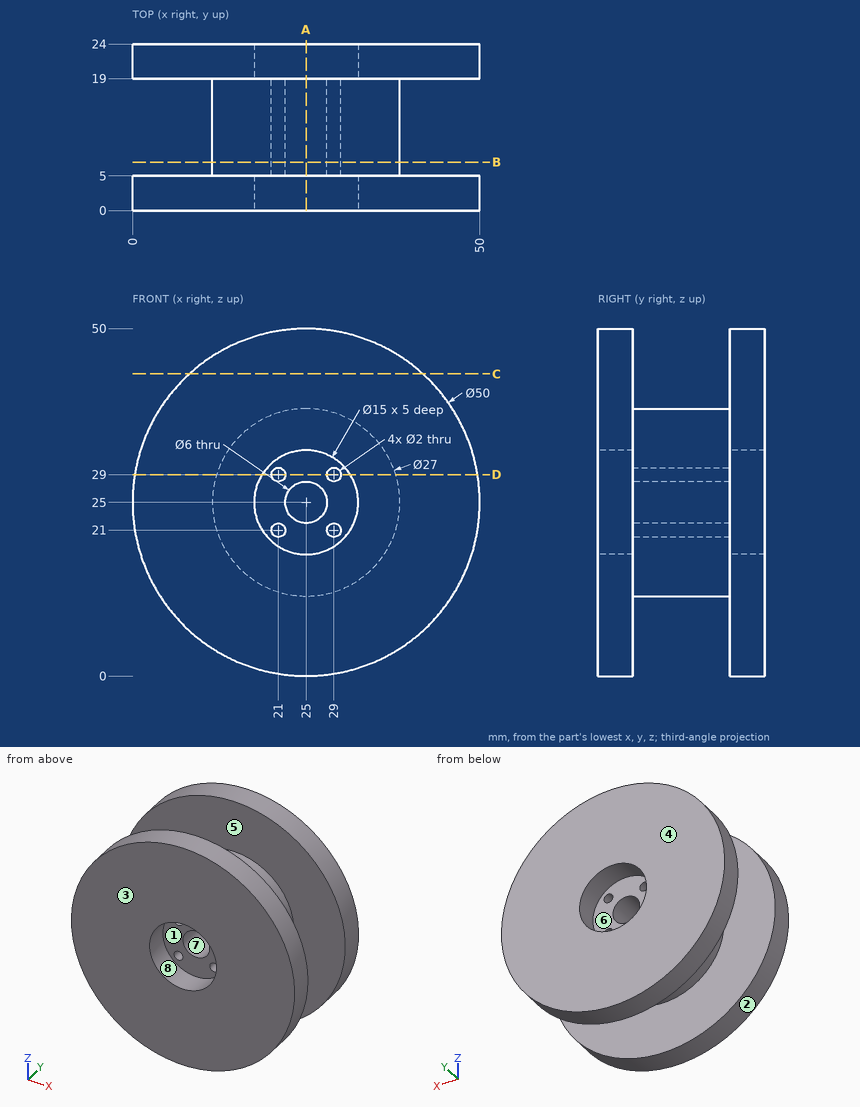
Design review of the part shown in the three views and the two pictorial views. Dimensions are in mm from the part's minimum x, y and z. A direction names the side the tool comes from. Round coordinates to 2 decimals unless told otherwise and drop trailing zeros. Order: outer loops, then holes, each group sorted by start corner. A loop starts at its lowest first (then second) coordinate and runs counter-clockwise, first axis right, second up.
Q1. Wall thickness on line 1 (Y direction, x = 38, z = 30); line 2 (X direction, y = 12.5, z = 25); line 3 (Z direction, x = 28.5, y = 12.25): over which ranges is each line inside the solid? List them lowest first.
Findings below:
line 1: y = 0 to 5, 19 to 24
line 2: x = 11.5 to 22, 28 to 38.5
line 3: z = 11.96 to 20.13, 21.87 to 28.13, 29.87 to 38.04
Q2. We need section B-B, the plane y = 7. Give the boundary of the cut face in (x, z).
Findings below:
outline: circle Ø27 at (25, 25); hole circle Ø2 at (21, 21); hole circle Ø2 at (21, 29); hole circle Ø6 at (25, 25); hole circle Ø2 at (29, 21); hole circle Ø2 at (29, 29)
Q3. We need section C-C, the plane z = 43.5. Give the boundary of the cut face in (x, y).
Findings below:
outline: (8.18, 0) - (41.82, 0) - (41.82, 5) - (8.18, 5) - close; (8.18, 19) - (41.82, 19) - (41.82, 24) - (8.18, 24) - close
Q4. Machinability: for the marked faces 4, 5, 6, 7 and 8, which of the approach directions +Z, -Z, +X, -X, +Y, -Y give a long, thin tool a straight path to every point of the face, cutting with its end or side? Answer none if there is none.
Findings below:
face 4: +Z, -Z, +X, -X, +Y
face 5: none
face 6: +Y
face 7: +Y, -Y
face 8: -Y
Q5. Mouldability with a two-part tool opening along X and no side actions: class the marked faces 1, 2 and 3 as pulls with the +X half, pulls with the -X half, needs draft (parallel to the pull), parting line crosses it, or undercut.
Findings below:
face 1: undercut
face 2: parting line crosses it
face 3: needs draft
Q6. Insertion check: P1, Ø3, axis at x = 20, z = 35, coming from the -Y side; P2, Ø8, axis at x = 10.5, y = 6, coming from the -Z side; P3, Ø2, axis at y = 14.5, z = 26, coming from the -X side; P4, Ø8, axis at x = 25, z = 25, coming from the +Y side. Each pin has a flat end and moves straight along its axis. Give the tip position at first contact, or say it passes through.
Findings below:
P1: stops at y = 0
P2: stops at z = 2.37
P3: stops at x = 11.5
P4: stops at y = 19
Q7. We need section A-A, the plane x = 25. Give the boundary of the cut face in (y, z).
Findings below:
outline: (0, 0) - (5, 0) - (5, 11.5) - (19, 11.5) - (19, 0) - (24, 0) - (24, 17.5) - (19, 17.5) - (19, 22) - (5, 22) - (5, 17.5) - (0, 17.5) - close; (0, 32.5) - (5, 32.5) - (5, 28) - (19, 28) - (19, 32.5) - (24, 32.5) - (24, 50) - (19, 50) - (19, 38.5) - (5, 38.5) - (5, 50) - (0, 50) - close
Q8. We need section D-D, the plane z = 29. Give the boundary of the cut face in (x, y).
Findings below:
outline: (0.32, 0) - (18.66, 0) - (18.66, 5) - (20, 5) - (20, 19) - (18.66, 19) - (18.66, 24) - (0.32, 24) - (0.32, 19) - (12.11, 19) - (12.11, 5) - (0.32, 5) - close; (22, 5) - (28, 5) - (28, 19) - (22, 19) - close; (30, 5) - (31.34, 5) - (31.34, 0) - (49.68, 0) - (49.68, 5) - (37.89, 5) - (37.89, 19) - (49.68, 19) - (49.68, 24) - (31.34, 24) - (31.34, 19) - (30, 19) - close
